Print and shaded views of the part. All mm, measured from the part's lowest x, y and z. A direction names the side the tool comes from. Give positions to 0.01 mm unless a question says otherwise; leave off trailing zeros. Write each loop counter-clockwise with the first axis right and the second up, starting at its lowest first coordinate (ties: lowest second). Pieces come first, ordered by that corner, then holes. Notation, with made-up numbers: (31, 53.5) -> (54, 53.5) arc R12 cw to (54, 62.5) -> close; hole circle Ø6 at (28, 33). An arc over 180 degrees is marked (long way). Put each result on its own line as item: value.
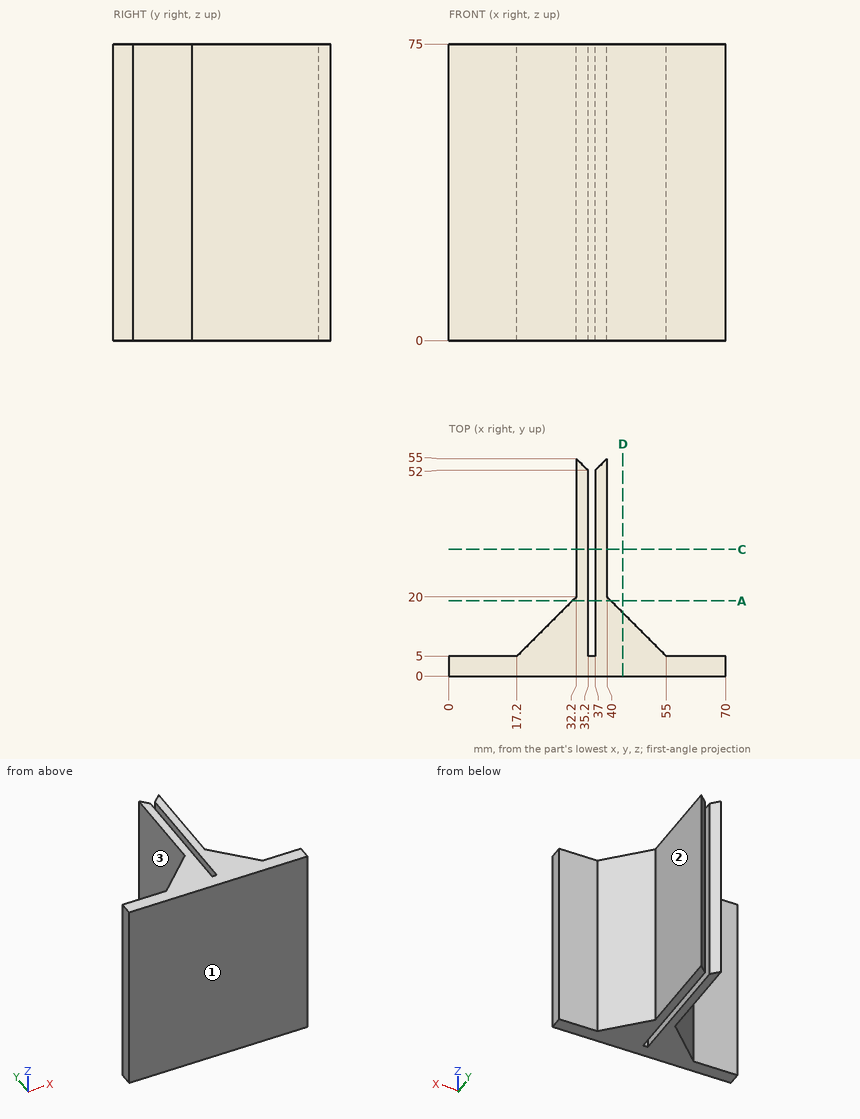
1) Slice it at A-A (y = 19). Write the cut outline in (x, z).
Filled sheet:
outline: (31.2, 0) -> (35.2, 0) -> (35.2, 75) -> (31.2, 75) -> close; (37, 0) -> (41, 0) -> (41, 75) -> (37, 75) -> close
2) Pin check, flat tips, straight feed: pin 1 (19 mm diameter, centred on x = 6, z = 45, fed in from +Y); pin 2 (1 mm diameter, centred on x = 43, z = 61.5, fed in from +Y); pin 3 (5 mm diameter, centred on x = 24.5, z = 54.5, fed in from -Y); pin 4 (16.5 mm diameter, centred on x = 59.5, z = 28, fed in from +Y). Stop position of each tip, or through.
Filled sheet:
pin 1: y = 5
pin 2: y = 17.5
pin 3: y = 0
pin 4: y = 8.75
3) Tool access for the marked faces 1, 2 and 3: list every direction of +Z, -Z, +X, -X, +Y, -Y with a clear straight run to the whole face (end or side of a thin tool).
Filled sheet:
face 1: +Z, -Z, +X, -X, -Y
face 2: +Z, -Z, +X, +Y
face 3: +Z, -Z, -X, +Y
4) Wall check: L1, parallel to X at y = 36.5, z = 60; L2, parallel to Y at x = 56.5, z = 50.5; L3, parallel to X at y = 16, z = 61. Give the ranges that are in metal, low to high.
Filled sheet:
L1: 32.2 to 35.2, 37 to 40
L2: 0 to 5
L3: 28.2 to 35.2, 37 to 44
5) Slice it at C-C (y = 32). Write the cut outline in (x, z).
Filled sheet:
outline: (32.2, 0) -> (35.2, 0) -> (35.2, 75) -> (32.2, 75) -> close; (37, 0) -> (40, 0) -> (40, 75) -> (37, 75) -> close
6) Slice it at D-D (x = 44). Write the cut outline in (y, z), plus the area to 3 significant figures.
Filled sheet:
outline: (0, 0) -> (16, 0) -> (16, 75) -> (0, 75) -> close
area: 1,200 mm2
